Can you work these out from the drawing? Everything is in mm from the part's minimum corner. Coordinates: 2 decimals unless noted, no trailing zeros. Order: outer loops, then holes, each group sorted by start corner. A loop starts at its lowest first (then second) coordinate and runs counter-clockwise, first axis right, second up. Notation, with made-up numbers: (36.5, 35) - (52.5, 35) arc R31 ccw to (52.5, 68) - close; hole circle Ø9 at (47, 54.5). An arc over 180 degrees is marked (long way). Use a Markdown table: item, result. Add a question column.
(1) I want a section at B-B (x = 330.2). List the corners of the cut face in (y, z) for me.
(2) For pin 1 Ø20 at (x, y) = (330.2, 25) entering from -Z, with a flat end and sliding along its axis, tell me the tip position at first contact or that it passes through.
(3) If I drill on L1, parallel to Y at x = 330.2, z = 3, over which ranges is the centre line in solid material (lowest first)? Write a range as [from, to].
(4) I want a section at A-A (y = 25). List the corners of the cut face in (x, z) for me, and give its area (3 significant figures).
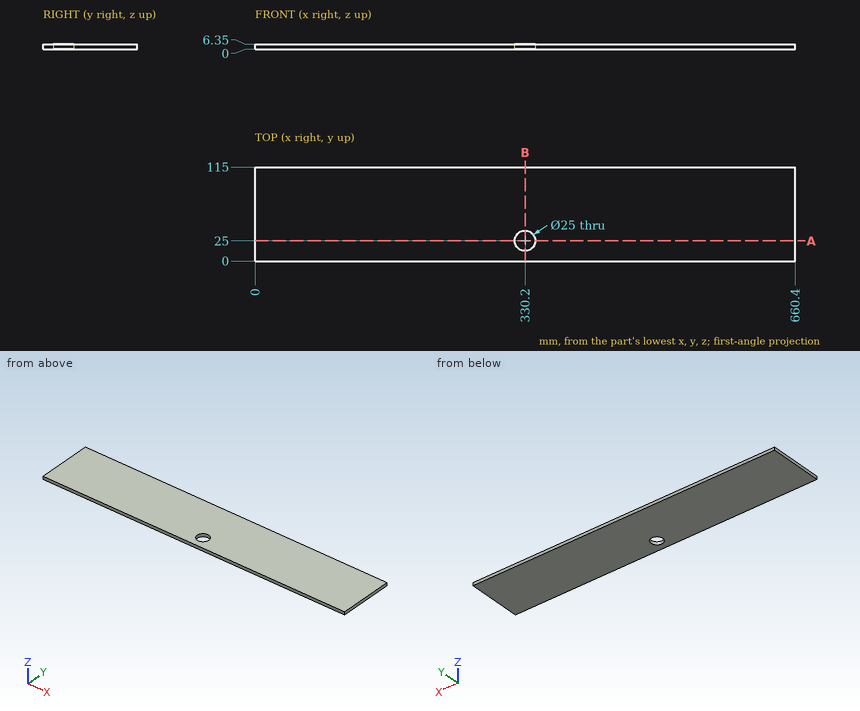
Answers follow:
| question | item | result |
|---|---|---|
| 1 | outline | (0, 0) - (12.5, 0) - (12.5, 6.35) - (0, 6.35) - close; (37.5, 0) - (115, 0) - (115, 6.35) - (37.5, 6.35) - close |
| 2 | pin 1 | passes through |
| 3 | L1 | y = [0, 12.5], [37.5, 115] |
| 4 | outline | (0, 0) - (317.7, 0) - (317.7, 6.35) - (0, 6.35) - close; (342.7, 0) - (660.4, 0) - (660.4, 6.35) - (342.7, 6.35) - close |
| 4 | area | 4,030 mm² |
